Verification items for the finished model (mm, model axes). A direction names the side the tool comes from. Give positions to 0.01 mm unless a question says otherwise; leave off trailing zeros. Write each loop counter-clockwise with the first axis right and the second up, starting at its lowest first coordinate (ties: lowest second). Pieces come first, ordered by that corner, then holes. Notation, with made-up numbers: (36.5, 30.5) -> (56.5, 30.5) arc R21 ccw to (56.5, 44.5) -> close; hole circle Ø1 at (35, -35.75). An arc over 180 degrees is marked (long way). Answer as CSV lines item,"result".
Autodesk Inventor part; units mm, degrees
ref_plane "YZ Plane" through (0, 0, 0) normal (1, 0, 0) x (0, 1, 0)
ref_plane "XZ Plane" through (0, 0, 0) normal (0, 1, 0) x (-1, 0, 0)
ref_plane "XY Plane" through (0, 0, 0) normal (0, 0, 1) x (1, 0, 0)
sketch "Sketch1" plane through (0, 0, 0) normal (1, 0, 0) x (0, 1, 0)
  circle A0 centre (12, -104.7) radius 4.375
  circle A1 centre (12, -104.7) radius 9 construction
  line L0 (12, -116.7) -> (12, -104.7) construction
  line L1 (12, -113.7) -> (12, -112.5)
  circle A2 centre (12, -112.5) radius 1.2
  circle A3 centre (12, -55.7) radius 2
  circle A4 centre (18.755, -108.6) radius 1.2
  circle A5 centre (18.755, -100.8) radius 1.2
  circle A6 centre (12, -96.9) radius 1.2
  circle A7 centre (5.245, -100.8) radius 1.2
  circle A8 centre (5.245, -108.6) radius 1.2
  line L2 (3, -43.2) -> (21, -43.2) construction
  line L3 (12, -116.7) -> (12, -71.7) construction
  line L4 (12, -71.7) -> (12, -63.7) construction
  line L5 (12, -63.7) -> (21, -63.7) construction
  line L6 (12, -63.7) -> (3, -63.7) construction
  line L7 (24, -72.7) -> (21, -63.7)
  line L8 (0, -71.7) -> (3, -63.7)
  line L9 (3, -43.2) -> (3, -63.7)
  line L10 (21, -43.2) -> (21, -63.7)
  arc A9 (24, 18.3) -> (0, 18.3) centre (12, 18.3) ccw
  circle A10 centre (12, -30.7) radius 2
  line L11 (12, -14.7) -> (12, -22.7) construction
  line L12 (12, -22.7) -> (21, -22.7) construction
  line L13 (12, -22.7) -> (3, -22.7) construction
  line L14 (24, -13.7) -> (21, -22.7)
  line L15 (0, -14.7) -> (3, -22.7)
  line L16 (3, -43.2) -> (3, -22.7)
  line L17 (0, 18.3) -> (0, -14.7)
  line L18 (24, 18.3) -> (24, -13.7)
  line L19 (21, -43.2) -> (21, -22.7)
  arc A11 (-3.3865, -101.1088) -> (27.3606, -100.9997) centre (12, -104.7) ccw
  line L20 (24, -72.7) -> (27.8, -104.7)
  line L21 (0, -71.7) -> (-3.8, -104.7)
  circle A12 centre (12, 18.3) radius 2
  point P0 (1.5, 26.1095)
  point P1 (22.5, 26.1095)
  point P2 (19.7942, -109.2)
  point P3 (19.7942, -100.2)
  point P4 (12, -95.7)
  point P5 (4.2058, -100.2)
  point P6 (4.2058, -109.2)
  dimension "d7" = 18
  dimension "d6" = 8.75
  dimension "d8" = 1.2
  dimension "d12" = 4
  dimension "d15" = 360
  dimension "d22" = 45
  dimension "d23" = 8
  dimension "d24" = 9
  dimension "d25" = 9
  dimension "d33" = 8
  dimension "d34" = 12.5
  dimension "d45" = 4
  dimension "d46" = 4
extrude "Extrusion2" add sketch "Sketch1" along normal blind 3 contours L20 A11 L21 L8 L9 L16 L15 L17 A9 L18 L14 L19 L10 L7
fillet "Face Fillet1" radius 10 1 edges at (1.5, 3, -22.7)
fillet "Face Fillet2" radius 10 1 edges at (1.5, 0, -14.7)
fillet "Face Fillet3" radius 10 1 edges at (1.5, 3, -63.7)
fillet "Face Fillet5" radius 10 1 edges at (1.5, 24, -13.7)
fillet "Face Fillet6" radius 10 1 edges at (1.5, 21, -22.7)
fillet "Face Fillet7" radius 10 1 edges at (1.5, 21, -63.7)
properties part number "Brazo1.1"
1) Section check B-B (z = -55.7). Record the boundary of the cut face in (x, y), and give its area (3 significant figures).
Reported:
outline,"(0, 3) -> (3, 3) -> (3, 10) -> (0, 10) -> close; (0, 14) -> (3, 14) -> (3, 21) -> (0, 21) -> close"
area,"42.0 mm²"
2) Section check C-C (z = -8.5). Record the boundary of the cut face in (x, y), and give its area (3 significant figures).
Reported:
outline,"(0, 0) -> (3, 0) -> (3, 24) -> (0, 24) -> close"
area,"72.0 mm²"
3) Depth check by flat-ended pin: pin 1 (3 mm diameter, centred on y = 12, z = -96.9, fed in from +X); pin 2 (0.9 mm diameter, centred on x = 1, z = -47, fed in from -Y); pin 3 (0.9 mm diameter, centred on x = 2, z = -43, fed in from +Y). Enter the tip coordinate at first touch or a pass-through.
Reported:
pin 1,"x = 3"
pin 2,"y = 3"
pin 3,"y = 21"
4) Section check D-D (y = 25.5). Record the boundary of the cut face in (x, z), and give its area (3 significant figures).
Reported:
outline,"(0, -112.91) -> (3, -112.91) -> (3, -85.33) -> (0, -85.33) -> close"
area,"82.7 mm²"
5) Tool access check on faces 1 (the flat face through (1, 0, 3)), 2 (the flat face through (1.479, 1.165, -68.593)), 3 (the flat face through (1, 21, -43)). Record the directions out of +Z, -Z, +X, -X, +Y, -Y that give a thin tool (end or side, any length) a straight path to the whole face; none if there is none.
Reported:
face 1,"+Z, +X, -X, -Y"
face 2,"+X, -X, -Y"
face 3,"+X, -X, +Y"
6) Section check A-A (x = 2.35). State how many separate pieces and enclosed holes the cut face has, and give its area (3 significant figures).
Reported:
separate pieces,"1"
enclosed holes,"10"
area,"3,270 mm²"
7) Draft check along Z on faces 4 (the flat face through (0, 12, -44)), 5 (the flat face through (1.5, 22.5, -18.2)), 6 (the cylindrical face through (1.479, 11.736, 30.297)). Enter one of: +Z half, -Z half, draft (parallel to the pull), parting line (faces both ways), or undercut.
Reported:
face 4,"draft"
face 5,"undercut"
face 6,"+Z half"
8) Scan lines: line 1 along Y through (x, z) = (2.85, -100); line 2 along Y through (x, z) = (1.05, -55.5); line 3 along Y through (x, z) = (0.15, 11.5). Record each from-to range of solid material in increasing order.
Reported:
line 1,"-3.26 to 4.35, 6.14 to 17.86, 19.65 to 27.24"
line 2,"3 to 10.01, 13.99 to 21"
line 3,"0 to 24"
